from build123d import *

# Parameters (mm, degrees)
F0_R     = 1.5934819676
F0_R_2   = 1.6180372771
F0_R_3   = 1.5947735427
F0_R_4   = 1.599183997
F0_R_5   = 1.5713503285
F0_R_6   = 1.584959903
F0_R_7   = 1.5945023752
F0_R_8   = 1.5875542678
F1_DEPTH = 3.175
F2_R     = 3.17499


# Not quite as in the source:
# - a fillet or chamfer is up to 0.001 mm smaller than in the source, because OpenCascade refuses the exact size


with BuildPart() as f1:
    # F0 (on Front) → F1 (new body)
    with BuildSketch(Plane.XZ):
        Polygon((64.607411623, 39.6379828453), (-62.5105649233, 39.6379828453), (0, -75.7666006684), align=None)
        with Locations((-5.3829359822, -53.0953221023)):
            Circle(F0_R, mode=Mode.SUBTRACT)
        with Locations((5.3829369135, -53.5846799612)):
            Circle(F0_R_2, mode=Mode.SUBTRACT)
        with Locations((-47.1807047725, 23.7195882946)):
            Circle(F0_R_3, mode=Mode.SUBTRACT)
        with Locations((-41.106056422, 32.5422920287)):
            Circle(F0_R_4, mode=Mode.SUBTRACT)
        with Locations((-6.8510090932, 33.5210077465)):
            Circle(F0_R_5, mode=Mode.SUBTRACT)
        with Locations((7.829724811, 33.5210077465)):
            Circle(F0_R_6, mode=Mode.SUBTRACT)
        with Locations((46.2791621685, 23.0933185667)):
            Circle(F0_R_7, mode=Mode.SUBTRACT)
        with Locations((40.1273407042, 31.5635800362)):
            Circle(F0_R_8, mode=Mode.SUBTRACT)
        with Locations((7.829724811, 33.5210077465)):
            Circle(F0_R_6)
        with Locations((-6.8510090932, 33.5210077465)):
            Circle(F0_R_5)
    extrude(amount=-F1_DEPTH)

    # F2 (radius 3.175 in the source; OpenCascade refuses exactly that, so slightly less here)
    f2_edges = [f1.edges().sort_by_distance(p)[0] for p in [
        (64.607412, 1.5875, 39.637983),
        (-62.510565, 1.5875, 39.637983),
        (0, 1.5875, -75.766601),
        (-31.255282, 0, -18.064309),
        (32.303706, 0, -18.064309),
        (1.048423, 0, 39.637983),
    ]]
    fillet(f2_edges, radius=F2_R)


solid = f1.part
Here's how the part is built. I have some questions about the finished solid (model axes, mm). Round coordinates to 2 decimals unless told otherwise and drop trailing zeros. Loops run counter-clockwise (first coordinate to the right, second up) from the corner with the lowest first, then second, coordinate; pieces in that order, holes last. Notation, with made-up numbers: (29, 50.25) - (66, 50.25) arc R23 ccw to (66, 70.25) - close; hole circle Ø3 at (-17.75, 53.5). An arc over 180 degrees is marked (long way). One line per question, with ' | ' between items. Start each with the question number.
Q1. Please list where these lines run through material, in increasing order: line 1 (Z direction, x = -48.5, y = 1.7); line 2 (Z direction, x = 47, y = 1.1); line 3 (X direction, y = 0.7, z = 19). Write a range as [from, to].
Q2. I want a section at A-A (y = 0.65). Write out the boundary of the cut face in (x, z), then the cut area to 3 significant figures.
Q3. We'd pull the mould along Z, two halves only. Please class faces 1 (the cylindrical face through (41.594, 1.565, 30.956)), 2 (the flat face through (0, 0, -4)), 3 (the cylindrical face through (32.01, 0.95, -16.73)): +Z half, -Z half, draft (parallel to the pull), parting line (faces both ways), or undercut.
Q4. Will these pins go through, and if not, where does the flat tip stop? pin 1 (1.9 mm diameter, centred on x = 5.38, z = -53.58, fed in from -Y); pin 2 (1.5 mm diameter, centred on y = 2, z = -16, fed in from -X).
Response values:
1) line 1: z = [14.54, 22.82], [24.62, 39.27] | line 2: z = [9.77, 21.67], [24.52, 38.87] | line 3: x = [-49.98, 51.69]
2) outline: (-58.87, 35.55) - (-1.65, -70.1) arc R1.92 ccw to (1.73, -70.13) - (60.87, 35.52) arc R1.92 ccw to (59.19, 38.39) - (-57.18, 38.39) arc R1.92 ccw to start; hole circle Ø3.19 at (-47.18, 23.72); hole circle Ø3.2 at (-41.11, 32.54); hole circle Ø3.19 at (-5.38, -53.1); hole circle Ø3.24 at (5.38, -53.58); hole circle Ø3.18 at (40.13, 31.56); hole circle Ø3.19 at (46.28, 23.09) | area: 6,800 mm²
3) face 1: undercut | face 2: draft | face 3: -Z half
4) pin 1: passes through | pin 2: stops at x = -32.61
